Geometry check sheet. Reference: the model listing, model coordinates, mm. Face numbers are marked on the shaded views. A direction names the side the tool comes from. Round coordinates to 2 decimals unless told otherwise and drop trailing zeros. Write each loop counter-clockwise with the first axis right and the second up, starting at its lowest first coordinate (ties: lowest second). Pieces come first, ordered by that corner, then holes. Notation, with made-up numbers: (80, 32) -> (108, 32) arc R22 cw to (108, 54) -> close; hole circle Ø3 at (82, 75.5). An arc over 180 degrees is marked (long way). Put each result on its own line as item: value. Start each with the question number.
from build123d import *

# Parameters (mm, degrees)
F1_R     = 25
F1_R_2   = 22.5
F1_R_3   = 15
F1_R_4   = 12.5
F2_DEPTH = 15
F3_R     = 5
F4_DEPTH = 11


with BuildPart() as f2:
    # F1 (on Front) → F2 (new body)
    with BuildSketch(Plane.XZ):
        Circle(F1_R)
        Circle(F1_R_2, mode=Mode.SUBTRACT)
        Circle(F1_R_3)
        Circle(F1_R_4, mode=Mode.SUBTRACT)
    extrude(amount=F2_DEPTH)

    # F3 (on offset) → F4 (join)
    with BuildSketch(Plane.XZ.offset(2)):
        with Locations((0, 19.220972)):
            Circle(F3_R)
        with Locations((-11.297804, 15.550093)):
            Circle(F3_R)
        with Locations((-18.280231, 5.939607)):
            Circle(F3_R)
        with Locations((-18.280231, -5.939607)):
            Circle(F3_R)
        with Locations((-11.297804, -15.550093)):
            Circle(F3_R)
        with Locations((0, -19.220972)):
            Circle(F3_R)
        with Locations((11.297804, -15.550093)):
            Circle(F3_R)
        with Locations((18.280231, -5.939607)):
            Circle(F3_R)
        with Locations((18.280231, 5.939607)):
            Circle(F3_R)
        with Locations((11.297804, 15.550093)):
            Circle(F3_R)
    extrude(amount=F4_DEPTH)


solid = f2.part
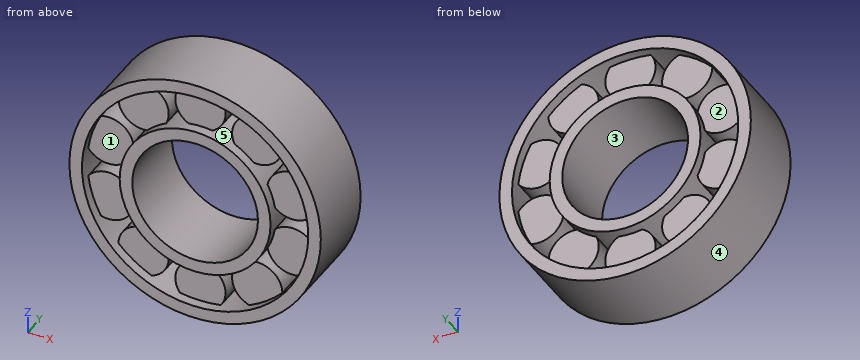
(1) Set-up check for the marked faces 1, 2 and 3: record each of +Z, -Z, +X, -X, +Y, -Y from which the full face is reachable in a straight line by a thin tool's end or side.
(2) Go/stop test with flat-tipped pins: pin 1 Ø4.5 at (x, z) = (-16, -8) entering from +Y; pin 2 Ø2 at (x, y) = (-13.5, -8) entering from +Z; pin 3 Ø5 at (y, z) = (-12.5, -5) entering from +X. Record where each tip stops, or that it passes through.
(3) Sectioned sample at C-C (y = -14). Record the cut outline in (x, z).
(4) Mould release check, pull along Z, two halves, no side actions. Record for the marked faces 4 and 5: +Z half, -Z half, draft (parallel to the pull), parting line (faces both ways), or undercut.
(5) Sectioned sample at B-B (x = 0). Record the cut outline in (y, z).
(6) Sectioned sample at A-A (z = 0). Record the cut outline in (x, y).
(7) Material ranges on L1, parallel to Z at x = -0.5, y = -13.25 (3 decimals); L2, parallel to Z at x = 0, y = -8; L3, parallel to Z at x = 7.5, y = -4.75, recorded low to high. Write a range as from..to.
(8) Sectioned sample at D-D (x = -8). Record the cut outline in (y, z), and give its area (3 significant figures).
Found:
1. face 1: -Y
1. face 2: +Y
1. face 3: +Y, -Y
2. pin 1: y = -2
2. pin 2: z = 21.65
2. pin 3: x = 24.87
3. outline: circle Ø50 at (0, 0); circle Ø30 at (0, 0); hole circle Ø45 at (0, 0); hole circle Ø25 at (0, 0)
4. face 4: parting line
4. face 5: undercut
5. outline: (-15, -25) -> (0, -25) -> (0, -22.5) -> (-2, -22.5) -> (-2, -15) -> (0, -15) -> (0, -12.5) -> (-15, -12.5) -> (-15, -15) -> (-13, -15) -> (-13, -22.5) -> (-15, -22.5) -> close; (-15, 12.5) -> (0, 12.5) -> (0, 15) -> (-2, 15) -> (-2, 22.5) -> (0, 22.5) -> (0, 25) -> (-15, 25) -> (-15, 22.5) -> (-13, 22.5) -> (-13, 15) -> (-15, 15) -> close
6. outline: (-25, -15) -> (-22.5, -15) -> (-22.5, 0) -> (-25, 0) -> close; (-15, -15) -> (-12.5, -15) -> (-12.5, 0) -> (-15, 0) -> close; (12.5, -15) -> (15, -15) -> (15, 0) -> (12.5, 0) -> close; (22.5, -15) -> (25, -15) -> (25, 0) -> (22.5, 0) -> close
7. L1: -24.995..-22.494, -14.992..-12.49, 12.49..14.992, 22.494..24.995
7. L2: -25..-12.5, 12.5..25
7. L3: -23.85..-21.21, -18.8..-10, 10..18.8, 21.21..23.85
8. outline: (-15, -23.69) -> (0, -23.69) -> (0, -21.03) -> (-15, -21.03) -> close; (-15, -12.69) -> (-13, -12.69) -> (-13, -19.31) -> (-2, -19.31) -> (-2, -12.69) -> (0, -12.69) -> (0, -9.6) -> (-15, -9.6) -> close; (-15, 9.6) -> (0, 9.6) -> (0, 12.69) -> (-2, 12.69) -> (-2, 19.31) -> (-13, 19.31) -> (-13, 12.69) -> (-15, 12.69) -> close; (-15, 21.03) -> (0, 21.03) -> (0, 23.69) -> (-15, 23.69) -> close
8. area: 318 mm2
